Could you check a few things on this model? Use its own coordinates, in mm. A direction names the side the tool comes from. Round coordinates to 2 decimals unless told otherwise and drop trailing zeros. Write each loop counter-clockwise with the first axis right and the second up, starting at its lowest first coordinate (ties: lowest second). Pieces come first, ordered by that corner, then holes. Notation, with made-up numbers: (5.25, 45) -> (29.25, 45) arc R36 cw to (29.25, 83) -> close; hole circle Ø4 at (44, 20). An arc over 180 degrees is marked (long way). Answer in a Markdown table with one row per item.
from build123d import *

# Parameters (mm, degrees)
BOSS_EXTRUDE1_DEPTH      = 65
BOSS_EXTRUDE1_DEPTH_BACK = 60
SKETCH3_W                = 20
SKETCH3_H                = 20
CUT_EXTRUDE1_DEPTH       = 1040.5


with BuildPart() as part:
    # Sketch1 → Boss-Extrude1 (new, two sides: drawn at the far end of the back side and taken through both)
    with BuildSketch(Plane(origin=(0, 0, 0), x_dir=(1, 0, 0), z_dir=(0, 1, 0)).offset(-BOSS_EXTRUDE1_DEPTH_BACK)):
        with BuildLine():
            Line((2.8, 0), (22.8, 0))
            ThreePointArc((22.8, 0), (24.779898987, -0.820101013), (25.6, -2.8))
            Line((25.6, -2.8), (25.6, -22.8))
            ThreePointArc((25.6, -22.8), (24.779898987, -24.779898987), (22.8, -25.6))
            Line((22.8, -25.6), (2.8, -25.6))
            ThreePointArc((2.8, -25.6), (0.820101013, -24.779898987), (0, -22.8))
            Line((0, -22.8), (0, -2.8))
            ThreePointArc((0, -2.8), (0.820101013, -0.820101013), (2.8, 0))
        make_face()
    extrude(amount=BOSS_EXTRUDE1_DEPTH + BOSS_EXTRUDE1_DEPTH_BACK)

    # Sketch3 → Cut-Extrude1 (cut)
    with BuildSketch(Plane(origin=(0, -60, 0), x_dir=(-1, 0, 0), z_dir=(0, -1, 0))):
        with Locations((-12.8, -12.8)):
            Rectangle(SKETCH3_W, SKETCH3_H)
    extrude(amount=-CUT_EXTRUDE1_DEPTH, mode=Mode.SUBTRACT)


solid = part.part
1) For faces 1 (the face through (13, 2, 2.8)), 2 (the face through (0, 2, 13)), which set-ups out of +Z, -Z, +X, -X, +Y, -Y let a thin tool reach every point of the face, with its end or its side?
Findings:
| item | result |
|---|---|
| face 1 | +Y, -Y |
| face 2 | +Z, -Z, -X, +Y, -Y |
2) Imagine slicing it at A-A, the plane y = -5. Please give me the cut outline in (x, z).
Findings:
| item | result |
|---|---|
| outline | (0, 2.8) arc R2.8 ccw to (2.8, 0) -> (22.8, 0) arc R2.8 ccw to (25.6, 2.8) -> (25.6, 22.8) arc R2.8 ccw to (22.8, 25.6) -> (2.8, 25.6) arc R2.8 ccw to (0, 22.8) -> close; hole (2.8, 2.8) -> (22.8, 2.8) -> (22.8, 22.8) -> (2.8, 22.8) -> close |
3) For pin 1 (10 mm diameter, centred on x = 4.5, z = 9, fed in from +Y), with a flat end and sliding along its axis, tell me the tip position at first contact or that it passes through.
Findings:
| item | result |
|---|---|
| pin 1 | stops at y = 65 |
4) Thinking about a two-plate mould opening in X: for faces 3 (the face through (2, -60, 13)), 4 (the face through (0.84, 1.62, 24.8)), 5 (the face through (13, 2, 22.8)), which applies, +X half, -X half, draft (parallel to the pull), parting line (faces both ways), or undercut?
Findings:
| item | result |
|---|---|
| face 3 | draft |
| face 4 | -X half |
| face 5 | undercut |
5) Imagine slicing it at D-D, the plane z = 24. Please give me the cut outline in (x, y).
Findings:
| item | result |
|---|---|
| outline | (0.27, -60) -> (25.33, -60) -> (25.33, 65) -> (0.27, 65) -> close |
6) Imagine slicing it at B-B, the plane z = 13.25. Please give me the cut outline in (x, y).
Findings:
| item | result |
|---|---|
| outline | (0, -60) -> (2.8, -60) -> (2.8, 65) -> (0, 65) -> close; (22.8, -60) -> (25.6, -60) -> (25.6, 65) -> (22.8, 65) -> close |
7) Please list where these lines run through material, in increasing order: line 1 (Z direction, x = 22.75, y = -6.5); line 2 (X direction, y = 2, z = 23.5).
Findings:
| item | result |
|---|---|
| line 1 | z = 0 to 2.8, 22.8 to 25.6 |
| line 2 | x = 0.09 to 25.51 |
8) Imagine slicing it at C-C, the plane x = 17.5. Please give me the cut outline in (y, z).
Findings:
| item | result |
|---|---|
| outline | (-60, 0) -> (65, 0) -> (65, 2.8) -> (-60, 2.8) -> close; (-60, 22.8) -> (65, 22.8) -> (65, 25.6) -> (-60, 25.6) -> close |
